Here's how the part is built. I have some questions about the finished solid (model axes, mm). A direction names the side the tool comes from. Give positions to 0.01 mm unless a question says otherwise; leave off trailing zeros. Loops run counter-clockwise (first coordinate to the right, second up) from the corner with the lowest first, then second, coordinate; pieces in that order, holes last. Notation, with made-up numbers: (42, 51) -> (55, 51) arc R8 ccw to (55, 65) -> close; hole circle Ø9 at (45, 83). An arc over 180 degrees is marked (long way). Answer in a Markdown table with one row per item. Add a question column.
Item 1: If we section it at C-C (x = -3): Write out the boundary of the cut face in (y, z), then the cut area to 3 significant figures.
Item 2: If we section it at A-A (z = 0.55): Write out the boundary of the cut face in (x, y), then the cut area to 3 significant figures.
Item 3: If I drill on line 1 (X direction, y = -0.8, z = 3.1); line 2 (Z direction, x = 0.5, y = -0.2); line 3 (Y direction, x = -0.25, z = 3.35), over which ranges is the centre line in solid material (lowest first)?
Item 4: We'd pull the mould along Y, two halves only. Please class faces 1 (the face through (-1, 3.36, 2)), 2 (the face through (-8, -0.24, 2)), 3 (the face through (-1, 1, 0)), 4 (the face through (-1, 1, 3.2)): released by +Y, released by -Y, zero draft, split by the parting line, or undercut.
Item 5: If we section it at B-B (y = 0.65): Write out the boundary of the cut face in (x, z).
Item 6: If we section it at D-D (x = 0.75): Write out the boundary of the cut face in (y, z), then the cut area to 3 significant figures.
Item 7: For P1, Ø0.8, axis at x = 6, z = 1, coming from the -Y side; P2, Ø2, axis at x = -2.5, y = 0.5, coming from the +Z side; P3, Ø0.5, axis at y = 2, z = 2, coming from the +X side; P4, Ø0.5, axis at x = -8, z = 1.5, coming from the +Y side, each with a flat end and sliding along its axis, tell me the tip position at first contact or that it passes through.
Item 8: Which directions (+Z, -Z, +X, -X, +Y, -Y) give clear straight access to the entire face, cutting with the end or side of a thin tool? Please do faces 5 (the face through (6, -0.23, 2)), 6 (the face through (5.503, 2, 2)), 7 (the face through (-8, 1.76, 2)).
```python
from build123d import *

# Parameters (mm, degrees)
F0_W     = 1.05921
F0_H     = 1.6
F0_W_2   = 1.05
F0_H_2   = 1.39079
F1_DEPTH = 3.2
F2_DEPTH = 3.6


with BuildPart() as f1:
    # F0 (on Top) → F1 (new body)
    with BuildSketch(Plane.XY):
        Polygon((6.352665, 1.360319), (6.352665, -0.030471), (5.302665, -0.030471), (5.302665, -0.230613), (5.502665, -0.230471), (6.552665, -0.230471), (6.552665, 1.560319), (5.502665, 1.560319), (5.302665, 1.563394), (5.302665, 1.360319), align=None)
        with BuildLine():
            Line((5.502665, -0.230471), (5.302665, -0.230613))
            Line((5.302665, -0.230613), (5.302665, -1.280471))
            ThreePointArc((5.302665, -1.280471), (5.138876, -1.675892), (4.743455, -1.839681))
            Line((4.743455, -1.839681), (-6.756545, -1.839681))
            ThreePointArc((-6.756545, -1.839681), (-7.145453, -1.67859), (-7.306545, -1.289681))
            Line((-7.306545, -1.289681), (-7.306545, -0.239539))
            Line((-7.306545, -0.239539), (-7.506545, -0.239681))
            Line((-7.506545, -0.239681), (-7.506545, -1.289681))
            ThreePointArc((-7.506545, -1.289681), (-7.286875, -1.820011), (-6.756545, -2.039681))
            Line((-6.756545, -2.039681), (4.743455, -2.039681))
            ThreePointArc((4.743455, -2.039681), (5.280298, -1.817314), (5.502665, -1.280471))
            Line((5.502665, -1.280471), (5.502665, -0.230471))
        make_face()
        Polygon((-7.506545, -0.239681), (-7.306545, -0.239539), (-7.306545, -0.039681), (-8.365755, -0.039681), (-8.365755, 1.560319), (-7.306545, 1.560319), (-7.306545, 1.757244), (-7.506545, 1.760319), (-8.565755, 1.760319), (-8.565755, -0.239681), align=None)
        with BuildLine():
            Line((5.302665, 2.610319), (5.302665, 1.563394))
            Line((5.302665, 1.563394), (5.502665, 1.560319))
            Line((5.502665, 1.560319), (5.502665, 2.610319))
            ThreePointArc((5.502665, 2.610319), (5.282995, 3.140649), (4.752665, 3.360319))
            Line((4.752665, 3.360319), (-6.756545, 3.360319))
            ThreePointArc((-6.756545, 3.360319), (-7.286875, 3.140649), (-7.506545, 2.610319))
            Line((-7.506545, 2.610319), (-7.506545, 1.760319))
            Line((-7.506545, 1.760319), (-7.306545, 1.757244))
            Line((-7.306545, 1.757244), (-7.306545, 2.610319))
            ThreePointArc((-7.306545, 2.610319), (-7.145453, 2.999228), (-6.756545, 3.160319))
            Line((-6.756545, 3.160319), (4.752665, 3.160319))
            ThreePointArc((4.752665, 3.160319), (5.141574, 2.999228), (5.302665, 2.610319))
        make_face()
        with BuildLine():
            Line((-7.306545, 1.757244), (5.302665, 1.563394))
            Line((5.302665, 1.563394), (5.302665, 2.610319))
            ThreePointArc((5.302665, 2.610319), (5.141574, 2.999228), (4.752665, 3.160319))
            Line((4.752665, 3.160319), (-6.756545, 3.160319))
            ThreePointArc((-6.756545, 3.160319), (-7.145453, 2.999228), (-7.306545, 2.610319))
            Line((-7.306545, 2.610319), (-7.306545, 1.757244))
        make_face()
        with Locations((-7.83615, 0.760319)):
            Rectangle(F0_W, F0_H)
        Polygon((5.302665, -0.230613), (5.302665, -0.030471), (5.302665, 1.360319), (5.302665, 1.563394), (-7.306545, 1.757244), (-7.306545, 1.560319), (-7.306545, -0.039681), (-7.306545, -0.239539), align=None)
        with BuildLine():
            Line((5.302665, -1.280471), (5.302665, -0.230613))
            Line((5.302665, -0.230613), (-7.306545, -0.239539))
            Line((-7.306545, -0.239539), (-7.306545, -1.289681))
            ThreePointArc((-7.306545, -1.289681), (-7.145453, -1.67859), (-6.756545, -1.839681))
            Line((-6.756545, -1.839681), (4.743455, -1.839681))
            ThreePointArc((4.743455, -1.839681), (5.138876, -1.675892), (5.302665, -1.280471))
        make_face()
        with Locations((5.827665, 0.664924)):
            Rectangle(F0_W_2, F0_H_2)
    extrude(amount=F1_DEPTH)

    # F0 (on Top) → F2 (join)
    with BuildSketch(Plane.XY):
        with BuildLine():
            Line((-7.306545, 1.757244), (5.302665, 1.563394))
            Line((5.302665, 1.563394), (5.302665, 2.610319))
            ThreePointArc((5.302665, 2.610319), (5.141574, 2.999228), (4.752665, 3.160319))
            Line((4.752665, 3.160319), (-6.756545, 3.160319))
            ThreePointArc((-6.756545, 3.160319), (-7.145453, 2.999228), (-7.306545, 2.610319))
            Line((-7.306545, 2.610319), (-7.306545, 1.757244))
        make_face()
        with BuildLine():
            Line((5.302665, -1.280471), (5.302665, -0.230613))
            Line((5.302665, -0.230613), (-7.306545, -0.239539))
            Line((-7.306545, -0.239539), (-7.306545, -1.289681))
            ThreePointArc((-7.306545, -1.289681), (-7.145453, -1.67859), (-6.756545, -1.839681))
            Line((-6.756545, -1.839681), (4.743455, -1.839681))
            ThreePointArc((4.743455, -1.839681), (5.138876, -1.675892), (5.302665, -1.280471))
        make_face()
        with BuildLine():
            Line((5.502665, -0.230471), (5.302665, -0.230613))
            Line((5.302665, -0.230613), (5.302665, -1.280471))
            ThreePointArc((5.302665, -1.280471), (5.138876, -1.675892), (4.743455, -1.839681))
            Line((4.743455, -1.839681), (-6.756545, -1.839681))
            ThreePointArc((-6.756545, -1.839681), (-7.145453, -1.67859), (-7.306545, -1.289681))
            Line((-7.306545, -1.289681), (-7.306545, -0.239539))
            Line((-7.306545, -0.239539), (-7.506545, -0.239681))
            Line((-7.506545, -0.239681), (-7.506545, -1.289681))
            ThreePointArc((-7.506545, -1.289681), (-7.286875, -1.820011), (-6.756545, -2.039681))
            Line((-6.756545, -2.039681), (4.743455, -2.039681))
            ThreePointArc((4.743455, -2.039681), (5.280298, -1.817314), (5.502665, -1.280471))
            Line((5.502665, -1.280471), (5.502665, -0.230471))
        make_face()
        with BuildLine():
            Line((5.302665, 2.610319), (5.302665, 1.563394))
            Line((5.302665, 1.563394), (5.502665, 1.560319))
            Line((5.502665, 1.560319), (5.502665, 2.610319))
            ThreePointArc((5.502665, 2.610319), (5.282995, 3.140649), (4.752665, 3.360319))
            Line((4.752665, 3.360319), (-6.756545, 3.360319))
            ThreePointArc((-6.756545, 3.360319), (-7.286875, 3.140649), (-7.506545, 2.610319))
            Line((-7.506545, 2.610319), (-7.506545, 1.760319))
            Line((-7.506545, 1.760319), (-7.306545, 1.757244))
            Line((-7.306545, 1.757244), (-7.306545, 2.610319))
            ThreePointArc((-7.306545, 2.610319), (-7.145453, 2.999228), (-6.756545, 3.160319))
            Line((-6.756545, 3.160319), (4.752665, 3.160319))
            ThreePointArc((4.752665, 3.160319), (5.141574, 2.999228), (5.302665, 2.610319))
        make_face()
    extrude(amount=F2_DEPTH)


solid = f1.part
```
Recorded:
| question | item | result |
|---|---|---|
| 1 | outline | (-2.04, 0) -> (3.36, 0) -> (3.36, 3.6) -> (1.69, 3.6) -> (1.69, 3.2) -> (-0.24, 3.2) -> (-0.24, 3.6) -> (-2.04, 3.6) -> close |
| 1 | area | 18.7 mm^2 |
| 2 | outline | (-8.57, -0.24) -> (-7.51, -0.24) -> (-7.51, -1.29) arc R0.75 ccw to (-6.76, -2.04) -> (4.74, -2.04) arc R0.76 ccw to (5.5, -1.28) -> (5.5, -0.23) -> (6.55, -0.23) -> (6.55, 1.56) -> (5.5, 1.56) -> (5.5, 2.61) arc R0.75 ccw to (4.75, 3.36) -> (-6.76, 3.36) arc R0.75 ccw to (-7.51, 2.61) -> (-7.51, 1.76) -> (-8.57, 1.76) -> close |
| 2 | area | 73.8 mm^2 |
| 3 | line 1 | x = -7.51 to 5.5 |
| 3 | line 2 | z = 0 to 3.2 |
| 3 | line 3 | y = -2.04 to -0.23, 1.65 to 3.36 |
| 4 | face 1 | released by +Y |
| 4 | face 2 | released by -Y |
| 4 | face 3 | zero draft |
| 4 | face 4 | undercut |
| 5 | outline | (-8.57, 0) -> (6.55, 0) -> (6.55, 3.2) -> (-8.57, 3.2) -> close |
| 6 | outline | (-2.04, 0) -> (3.36, 0) -> (3.36, 3.6) -> (1.63, 3.6) -> (1.63, 3.2) -> (-0.23, 3.2) -> (-0.23, 3.6) -> (-2.04, 3.6) -> close |
| 6 | area | 18.7 mm^2 |
| 7 | P1 | stops at y = -0.23 |
| 7 | P2 | stops at z = 3.6 |
| 7 | P3 | stops at x = 5.5 |
| 7 | P4 | stops at y = 1.76 |
| 8 | face 5 | +Z, -Z, +X, -Y |
| 8 | face 6 | +Z, -Z, +X, +Y |
| 8 | face 7 | +Z, -Z, -X, +Y |
